```python
from build123d import *

# Parameters (mm, degrees)
CUT_EXTRUDE1_DEPTH = 5.08


with BuildPart() as part:
    # Sketch1 → Loft1 section 0
    with BuildSketch(Plane(origin=(0, 0, 0), x_dir=(1, 0, 0), z_dir=(0, 1, 0))):
        with BuildLine():
            Line((0, 0), (12.7, 0))
            Line((12.7, 0), (12.7, 3.175))
            Line((12.7, 3.175), (0, 3.175))
            Line((0, 3.175), (0, 0))
        make_face()
    # Sketch2 → Loft1 section 1
    with BuildSketch(Plane(origin=(0, 432.562, 0), x_dir=(1, 0, 0), z_dir=(0, 1, 0))):
        with BuildLine():
            Line((77.47, 0), (90.17, 0))
            Line((90.17, 0), (90.17, 3.175))
            Line((90.17, 3.175), (77.47, 3.175))
            Line((77.47, 3.175), (77.47, 0))
        make_face()
    loft()

    # Sketch3 → Cut-Extrude1 (cut)
    with BuildSketch(Plane.XY):
        Polygon((83.541818167, 432.562), (83.541818167, 429.26), (89.578625954, 429.26), (90.17, 432.562), align=None)
        Polygon((6.071818167, 3.175), (6.071818167, 0), (12.7, 0), (13.26862889, 3.175), align=None)
        Polygon((26.699924676, 117.475), (26.699924676, 114.3), (33.170640047, 114.3), (33.739268937, 117.475), align=None)
        Polygon((69.331344794, 353.695), (69.331344794, 350.52), (75.476629477, 350.52), (76.045258368, 353.695), align=None)
        Polygon((55.120871422, 274.955), (55.120871422, 271.78), (61.374633001, 271.78), (61.943261891, 274.955), align=None)
        Polygon((40.910398049, 193.04), (40.910398049, 196.215), (47.841265414, 196.215), (47.272636524, 193.04), align=None)
    extrude(amount=-CUT_EXTRUDE1_DEPTH, mode=Mode.SUBTRACT)


solid = part.part
```
Check sheet for the modelled part. Datum: model origin and axes. Units: mm. Round coordinates to 2 decimals unless told otherwise and drop trailing zeros. Loops run counter-clockwise (first coordinate to the right, second up) from the corner with the lowest first, then second, coordinate; pieces in that order, holes last. Notation, with made-up numbers: (75, 79) -> (102, 79) arc R23 ccw to (102, 97) -> close; hole circle Ø1 at (-14, 33). An arc over 180 degrees is marked (long way). Answer in a Markdown table with one row per item.
Q1. Go/stop test with flat-tipped pins: P1, Ø1, axis at y = 177.5, z = -2.5, coming from the -X side; P2, Ø1, axis at y = 116, z = -1.5, coming from the +X side; P3, Ø1.6, axis at y = 273, z = -1, coming from the +X side. Record where each tip stops, or that it passes through.
Data:
| item | result |
|---|---|
| P1 | stops at x = 31.7 |
| P2 | stops at x = 26.7 |
| P3 | stops at x = 55.12 |
Q2. Sectioned sample at A-A on z = -0.6. Enter the section's corners in (x, y) (3 decimals).
Data:
| item | result |
|---|---|
| outline | (0, 0) -> (6.072, 0) -> (6.072, 3.175) -> (13.269, 3.175) -> (33.171, 114.3) -> (26.7, 114.3) -> (26.7, 117.475) -> (33.739, 117.475) -> (47.273, 193.04) -> (40.91, 193.04) -> (40.91, 196.215) -> (47.841, 196.215) -> (61.375, 271.78) -> (55.121, 271.78) -> (55.121, 274.955) -> (61.943, 274.955) -> (75.477, 350.52) -> (69.331, 350.52) -> (69.331, 353.695) -> (76.045, 353.695) -> (89.579, 429.26) -> (83.542, 429.26) -> (83.542, 432.562) -> (77.47, 432.562) -> close |
Q3. Thickness scan on L1, parallel to X at y = 325, z = -2.35; L2, parallel to X at y = 135.5, z = -0.35. Record the ranges inside material, lowest first.
Data:
| item | result |
|---|---|
| L1 | x = 58.21 to 70.91 |
| L2 | x = 24.27 to 36.97 |
